```python
from build123d import *

# Parameters (mm, degrees)
F0_R     = 10.5
F1_DEPTH = 290
F2_R     = 7
F3_DEPTH = 300
F5_W     = 300
F5_H     = 10
F6_DEPTH = 25
F8_DEPTH = 25


with BuildPart() as f1:
    # F0 (on Right) → F1 (new body)
    with BuildSketch(Plane.YZ):
        Circle(F0_R)
    extrude(amount=F1_DEPTH)

    # F2 (on face) → F3 (cut)
    with BuildSketch(Plane(origin=(0, 0, 0), x_dir=(0, -1, 0), z_dir=(-1, 0, 0))):
        Circle(F2_R)
    extrude(amount=-F3_DEPTH, mode=Mode.SUBTRACT)

    # F5 (on Top) → F6 (cut)
    with BuildSketch(Plane.XY):
        Rectangle(F5_W, F5_H)
    extrude(amount=F6_DEPTH, mode=Mode.SUBTRACT)

    # F7 (on Top) → F8 (cut)
    with BuildSketch(Plane.XY):
        with BuildLine():
            ThreePointArc((14, 0), (12, 2), (10, 0))
            Line((10, 0), (12, 0))
            Line((12, 0), (14, 0))
        make_face()
        with BuildLine():
            ThreePointArc((238, 0), (236, 2), (234, 0))
            ThreePointArc((234, 0), (236, -2), (238, 0))
        make_face()
        with BuildLine():
            ThreePointArc((145, 0), (143, 2), (141, 0))
            Line((141, 0), (143, 0))
            Line((143, 0), (145, 0))
        make_face()
        with BuildLine():
            Line((143, 0), (141, 0))
            ThreePointArc((141, 0), (143, -2), (145, 0))
            Line((145, 0), (143, 0))
        make_face()
        with BuildLine():
            Line((12, 0), (10, 0))
            ThreePointArc((10, 0), (12, -2), (14, 0))
            Line((14, 0), (12, 0))
        make_face()
    extrude(amount=-F8_DEPTH, mode=Mode.SUBTRACT)


solid = f1.part
```
The model under review builds one solid part; all positions refer to its coordinate system, in mm. A direction names the side the tool comes from. Give positions to 0.01 mm unless a question says otherwise; leave off trailing zeros. Write each loop counter-clockwise with the first axis right and the second up, starting at its lowest first coordinate (ties: lowest second). Pieces come first, ordered by that corner, then holes. Notation, with made-up numbers: (56.25, 59) -> (90.25, 59) arc R31 cw to (90.25, 86) -> close; hole circle Ø11 at (-7.5, 16.5). An arc over 180 degrees is marked (long way). Answer in a Markdown table with one row per item.
1) Tool access review of faces 4 (the flat face through (290, 2, -7)), 5 (the flat face through (150, 0, 8)): name each direction out of +Z, -Z, +X, -X, +Y, -Y from which nothing blocks a thin tool from reaching the whole face with its end or side.
Worked answers:
| item | result |
|---|---|
| face 4 | +Z, -Z, +X, +Y, -Y |
| face 5 | +Z, -X |
2) Mouldability with a two-part tool opening along Y and no side actions: class faces 1 (the flat face through (0, 2, -7)), 2 (the cylindrical face through (142.97, -3.23, -6.21)), 3 (the cylindrical face through (142.97, 4.845, -9.315)) as +Y half, -Y half, draft (parallel to the pull), parting line (faces both ways), or undercut.
Worked answers:
| item | result |
|---|---|
| face 1 | draft |
| face 2 | undercut |
| face 3 | parting line |
3) Add section A-A on x = 254.5. State the section outline as (y, z) points, plus the area to 3 significant figures.
Worked answers:
| item | result |
|---|---|
| outline | circle Ø21 at (0, 0); hole circle Ø14 at (0, 0) |
| area | 192 mm² |
4) Clearance check with flat-ended pins moving along their axes: P1, Ø1.3, axis at x = 39.5, z = 7, coming from the +Y side; P2, Ø3, axis at y = 1.5, z = 8.5, coming from the -X side; P3, Ø5, axis at x = 143, y = 0, coming from the +Z side; P4, Ø2, axis at y = -5, z = 0, coming from the -X side. State where each tip first meets the part, or that it passes through.
Worked answers:
| item | result |
|---|---|
| P1 | y = 8.36 |
| P2 | x = 150 |
| P3 | z = -6.54 |
| P4 | through |
5) Add section B-B on x = 60.5. State the section outline as (y, z) points, plus the area to 3 significant figures.
Worked answers:
| item | result |
|---|---|
| outline | (-5, 4.9) -> (-5, 9.23) arc R10.5 ccw (long way) to (5, 9.23) -> (5, 4.9) arc R7 cw (long way) to start |
| area | 155 mm² |
6) For L1, parallel to Y at x = 183.5, z = 0; L2, parallel to Y at x = 64.5, z = 8, list the stretches that pass through material, from the lowest coordinate up. Write a range as [from, to].
Worked answers:
| item | result |
|---|---|
| L1 | [-10.5, -7], [7, 10.5] |
| L2 | [-6.8, -5], [5, 6.8] |
